Could you check a few things on this model? Use its own coordinates, in mm. Give positions to 0.01 mm unless a question says otherwise; leave off trailing zeros. Order: outer loops, then holes, each group sorted by start corner. A loop starts at its lowest first (then second) coordinate and runs counter-clockwise, first axis right, second up.
Autodesk Inventor part; units mm, degrees
ref_plane "Work Plane2" through (0, -4, 0) normal (0, 1, 0) x (-1, 0, 0)
ref_plane "YZ Plane" through (0, 0, 0) normal (1, 0, 0) x (0, 1, 0)
ref_plane "XY Plane" through (0, 0, 0) normal (0, 0, 1) x (1, 0, 0)
sketch "Sketch1" plane through (0, 0, 0) normal (1, 0, 0) x (0, 1, 0)
  circle A0 centre (0, 0) radius 4
  dimension "d0" = 8
extrude "Extrusion1" add sketch "Sketch1" along normal blind 200
sketch "Sketch2" plane through (0, 0, 0) normal (0, 1, 0) x (-1, 0, 0)
  line L0 (0, 0) -> (-15, 0)
  line L1 (-15, 0) -> (-30, 0)
  circle A0 centre (-30, 0) radius 2.5
  circle A1 centre (-15, 0) radius 2.5
  dimension "d3" = 15
  dimension "d4" = 15
  dimension "d5" = 5
  dimension "d6" = 5
extrude "Extrusion2" cut sketch "Sketch2" along normal mid plane 200
sketch "Sketch3" plane through (200, 0, 0) normal (1, 0, 0) x (0, 0, -1)
  circle A0 centre (0, 0) radius 3
  dimension "d9" = 6
extrude "Extrusion3" cut sketch "Sketch3" against normal blind 20
thread "Thread1"
ref_plane "Work Plane2" through (0, -4, 0) normal (0, 1, 0) x (-1, 0, 0)
sketch "Sketch4" plane through (0, -4, 0) normal (0, 1, 0) x (-1, 0, 0)
  line L0 (0, 4) -> (0, -4)
  line L1 (0, -4) -> (-200, -4)
  line L2 (0, 4) -> (-40, 4)
  line L3 (-40, 4) -> (-40, -4)
  line L4 (-40, -4) -> (0, -4)
  line L5 (0, -4) -> (0, 4)
  point P0 (0, 0)
  dimension "d16" = 40
extrude "Extrusion4" cut sketch "Sketch4" along normal blind 0.5
properties part number "counterweight-rod" material "Aluminum 6061"
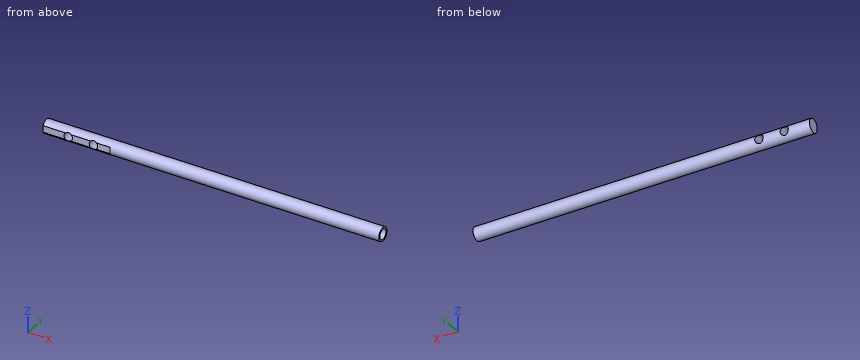
Item 1: Please list where these lines run through material, in increasing order: line 1 along X through (y, z) = (0.5, 0); line 2 along Z through (x, y) = (15, 0); line 3 along X through (y, z) = (1.75, -0.5).
Findings:
line 1: x = 0 to 12.5, 17.5 to 27.5, 32.5 to 180
line 2: z = -4 to -2.5, 2.5 to 4
line 3: x = 0 to 12.55, 17.45 to 27.55, 32.45 to 180
Item 2: For pin 1 (1.9 mm diameter, centred on x = 4, z = 0.5, fed in from -Y); pin 2 (2 mm diameter, centred on x = 46, y = 1, fed in from +Z); pin 3 (1 mm diameter, centred on x = 21.5, y = 2.5, fed in from +Z); pin 4 (1 mm diameter, centred on x = 56, z = -3, fed in from -Y), each with a flat end and sliding along its axis, tell me the tip position at first contact or that it passes through.
Findings:
pin 1: stops at y = -3.5
pin 2: stops at z = 4
pin 3: stops at z = 3.46
pin 4: stops at y = -3.12
Item 3: Imagine slicing it at A-A on y = 0. List the corners of the cut face in (x, z) for me, then the cut area to 3 significant figures.
Findings:
outline: (0, -4) - (200, -4) - (200, -3) - (180, -3) - (180, 3) - (200, 3) - (200, 4) - (0, 4) - close; hole circle Ø5 at (15, 0); hole circle Ø5 at (30, 0)
area: 1,440 mm2
Item 4: Imagine slicing it at B-B on x = 176.5. List the corners of the cut face in (y, z) for me.
Findings:
outline: circle Ø8 at (0, 0)
